Design review of the part built by this model. Coordinates are the model's own, in mm. Coordinates: 2 decimals unless noted, no trailing zeros. Loops run counter-clockwise (first coordinate to the right, second up) from the corner with the lowest first, then second, coordinate; pieces in that order, holes last. Notation, with made-up numbers: M 10,-30.5 L 46,-30.5 A23 ccw 46,3.5 Z; hole C 19.25,78 d7. An arc over 180 degrees is marked long. Write item = value, one per line. Start each with the question number.
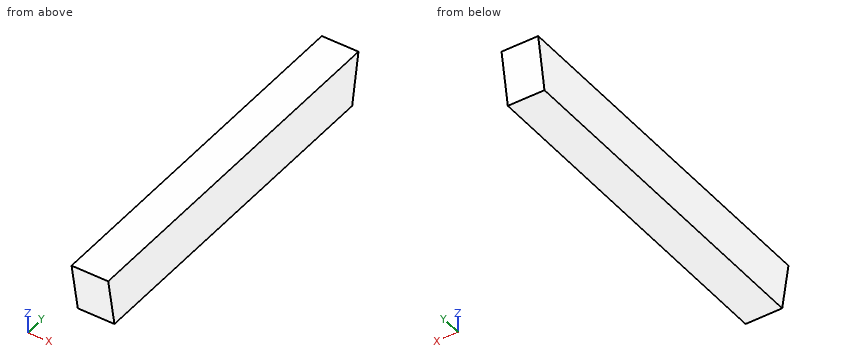
```python
from build123d import *

# Parameters (mm, degrees)
F0_W     = 20
F0_H     = 28
F1_DEPTH = 200
F2_SIZE2 = 27.99999
F2_SIZE  = 4.99999
F3_SIZE2 = 4.99999
F3_SIZE  = 27.99999


# Not quite as in the source:
# - a fillet or chamfer is up to 0.001 mm smaller than in the source, because OpenCascade refuses the exact size


with BuildPart() as f1:
    # F0 (on Front) → F1 (new body)
    with BuildSketch(Plane.XZ):
        Rectangle(F0_W, F0_H)
    extrude(amount=F1_DEPTH)

    # F2 (size 5 and 28 in the source; OpenCascade refuses exactly that, so slightly less here)
    f2_edges = [f1.edges().sort_by_distance(p)[0] for p in [
        (0, -200, -14),
    ]]
    f2_side = f1.faces().sort_by_distance((0, -100, -14))[0]
    chamfer(f2_edges, length=F2_SIZE, length2=F2_SIZE2, reference=f2_side)

    # F3 (size 28 and 5 in the source; OpenCascade refuses exactly that, so slightly less here)
    f3_edges = [f1.edges().sort_by_distance(p)[0] for p in [
        (0, 0, -14),
    ]]
    f3_side = f1.faces().sort_by_distance((0, 0, 0))[0]
    chamfer(f3_edges, length=F3_SIZE, length2=F3_SIZE2, reference=f3_side)


solid = f1.part
```
(1) Insertion check: pin 1 (4 mm diameter, centred on x = 3.5, z = 6, fed in from +Y); pin 2 (3 mm diameter, centred on x = -6, z = 5.5, fed in from +Y); pin 3 (8 mm diameter, centred on x = 6, z = 7, fed in from +Y). Each pin has a flat end and moves straight along its axis. Give the tip position at first contact, or say it passes through.
(2) To check wall thickness, follow L1, parallel to Y at x = 9.25, z = 4.5; L2, parallel to Y at x = -5.5, z = 1.25. State the ranges of each line that lie inside material, in increasing order.
(3) Take a section at B-B (z = -0.75). State the section outline as (x, y) points, plus the area to 3 significant figures.
Results list:
q1.pin_1 = -1.07
q1.pin_2 = -1.25
q1.pin_3 = -0.54
q2.L1 = -198.3 to -1.7
q2.L2 = -197.72 to -2.28
q3.outline = M -10,-197.37 L 10,-197.37 L 10,-2.63 L -10,-2.63 Z
q3.area = 3,890 mm^2
